from build123d import *

# Parameters (mm, degrees)
F1_DEPTH       = 15
F3_D           = 5
F3_DEPTH       = 11
F3_CSINK_D     = 9
F3_CSINK_ANGLE = 90
F4_R           = 5
F5_R           = 3


with BuildPart() as f1:
    # F0 (on Top) → F1 (new body)
    with BuildSketch(Plane.XY):
        Polygon((0, -25.4), (0, 0), (68.63, 0), (68.63, -25.4), (61.63, -25.4), (61.63, -28.4), (71.63, -28.4), (71.63, 3), (-3, 3), (-3, -28.4), (7, -28.4), (7, -25.4), align=None)
    extrude(amount=F1_DEPTH)

    # F3
    with Locations(Plane.XZ):
        with Locations((34.315, 7.5)):
            CounterSinkHole(F3_D / 2, F3_CSINK_D / 2, depth=F3_DEPTH, counter_sink_angle=F3_CSINK_ANGLE)

    # F4
    f4_edges = [f1.edges().sort_by_distance(p)[0] for p in [
        (7, -26.9, 15),
        (61.63, -26.9, 15),
        (7, -26.9, 0),
        (61.63, -26.9, 0),
    ]]
    fillet(f4_edges, radius=F4_R)

    # F5
    f5_edges = [f1.edges().sort_by_distance(p)[0] for p in [
        (0, -25.4, 7.5),
        (-3, -28.4, 7.5),
        (71.63, -28.4, 7.5),
        (68.63, -25.4, 7.5),
    ]]
    fillet(f5_edges, radius=F5_R)


solid = f1.part
Build history of the part. All positions in model axes, mm. A direction names the side the tool comes from. Give positions to 0.01 mm unless a question says otherwise; leave off trailing zeros. Loops run counter-clockwise (first coordinate to the right, second up) from the corner with the lowest first, then second, coordinate; pieces in that order, holes last. Notation, with made-up numbers: (19, -27.75) -> (70, -27.75) arc R31 ccw to (70, -3.75) -> close; hole circle Ø5 at (87.5, 76.5). An arc over 180 degrees is marked (long way). Answer in a Markdown table with one row per item.
Item 1: Slice it at A-A on z = 7.5. Write the cut outline in (x, y) (3 decimals).
Findings below:
| item | result |
|---|---|
| outline | (-3, -25.4) arc R3 ccw to (0, -28.4) -> (7, -28.4) -> (7, -25.4) -> (3, -25.4) arc R3 cw to (0, -22.4) -> (0, 0) -> (29.815, 0) -> (31.815, 2) -> (31.815, 3) -> (-3, 3) -> close; (36.815, 2) -> (38.815, 0) -> (68.63, 0) -> (68.63, -22.4) arc R3 cw to (65.63, -25.4) -> (61.63, -25.4) -> (61.63, -28.4) -> (68.63, -28.4) arc R3 ccw to (71.63, -25.4) -> (71.63, 3) -> (36.815, 3) -> close |
Item 2: Slice it at C-C on z = 14. Write the cut outline in (x, y), plus the area to 3 significant figures.
Findings below:
| item | result |
|---|---|
| outline | (-3, -25.4) arc R3 ccw to (0, -28.4) -> (5, -28.4) -> (5, -25.4) -> (3, -25.4) arc R3 cw to (0, -22.4) -> (0, 0) -> (68.63, 0) -> (68.63, -22.4) arc R3 cw to (65.63, -25.4) -> (63.63, -25.4) -> (63.63, -28.4) -> (68.63, -28.4) arc R3 ccw to (71.63, -25.4) -> (71.63, 3) -> (-3, 3) -> close |
| area | 424 mm² |
Item 3: Mould opens along X. For faces 4 (the cylindrical face through (70.73, -27.54, 7.6)), 5 (the cylindrical face through (67.73, -24.54, 7.6)), 6 (the flat face through (35, 3, 4)) say: pulls with the +X half, pulls with the -X half, needs draft (parallel to the pull), parting line crosses it, or undercut.
Findings below:
| item | result |
|---|---|
| face 4 | pulls with the +X half |
| face 5 | undercut |
| face 6 | needs draft |
Item 4: Slice it at D-D on x = 17. Write the cut outline in (y, z), plus the area to 3 significant figures.
Findings below:
| item | result |
|---|---|
| outline | (0, 0) -> (3, 0) -> (3, 15) -> (0, 15) -> close |
| area | 45.0 mm² |
Item 5: Slice it at B-B on y = -20.5. Write the cut outline in (x, z).
Findings below:
| item | result |
|---|---|
| outline | (-3, 0) -> (0, 0) -> (0, 15) -> (-3, 15) -> close; (68.63, 0) -> (71.63, 0) -> (71.63, 15) -> (68.63, 15) -> close |
Item 6: Probe line 1 along Y through (x, z) = (64, 13.5); line 2 along X through (y, z) = (2.55, 7.5) (3 decimals); line 3 along X through (y, z) = (-20, 4.5). List the from-to ranges inside material, lowest first. Write a range as [from, to].
Findings below:
| item | result |
|---|---|
| line 1 | y = [-28.4, -25.4], [0, 3] |
| line 2 | x = [-3, 31.815], [36.815, 71.63] |
| line 3 | x = [-3, 0], [68.63, 71.63] |
Item 7: Tool access for faces 1 (the flat face through (7, -27, 7)), 2 (the cylindrical face through (63.13, -26.84, 13.57)), 3 (the flat face through (68.63, -11, 7)): list every direction of +Z, -Z, +X, -X, +Y, -Y with a clear straight run to the whole face (end or side of a thin tool).
Findings below:
| item | result |
|---|---|
| face 1 | +Z, -Z, -Y |
| face 2 | +Z, -Y |
| face 3 | +Z, -Z |
Item 8: Flat gauge pins, fed straight in: P1, Ø1.5, axis at y = -27.5, z = 8.5, coming from the -X side; P2, Ø3, axis at x = 28, z = 5, coming from the -Y side; P3, Ø0.9, axis at y = -26, z = 6.5, coming from the +X side. Where does each tip first touch, or does it go through?
Findings below:
| item | result |
|---|---|
| P1 | stops at x = -2.68 |
| P2 | stops at y = 0 |
| P3 | stops at x = 71.63 |
